For this review, take the finished solid that the model builds, in its own axes (mm). A direction names the side the tool comes from. Round coordinates to 2 decimals unless told otherwise and drop trailing zeros. Loops run counter-clockwise (first coordinate to the right, second up) from the corner with the lowest first, then second, coordinate; pieces in that order, holes last.
```python
from build123d import *

# Parameters (mm, degrees)
EXTRUDE_1_DEPTH      = 38
EXTRUDE_1_DEPTH_BACK = 38
EXTRUDE_2_DEPTH      = 60
SKETCH_4_R           = 1.5
SKETCH_4_W           = 14
SKETCH_4_H           = 18
CUT_EXTRUDE_1_DEPTH  = 6
CUT_EXTRUDE_3_DEPTH  = 14
FILLET_2_R           = 3
CUT_EXTRUDE_6_DEPTH  = 3
SKETCH_13_R          = 1.5
CUT_EXTRUDE_7_DEPTH  = 10
CUT_EXTRUDE_9_DEPTH  = 15
SKETCH_17_W          = 41
SKETCH_17_H          = 26
SKETCH_17_R          = 9.5
SKETCH_17_R_2        = 1.5
EXTRUDE_3_DEPTH      = 3
FILLET_3_R           = 10
SKETCH_18_W          = 17
SKETCH_18_H          = 40
CUT_EXTRUDE_10_DEPTH = 10
FILLET_4_R           = 8
CUT_EXTRUDE_11_DEPTH = 4
FILLET_5_R           = 1
CUT_EXTRUDE_12_DEPTH = 10


with BuildPart() as part:
    # Sketch 2 → Extrude 1 (new, two sides: drawn at the far end of the back side and taken through both)
    with BuildSketch(Plane.XY.offset(-EXTRUDE_1_DEPTH_BACK)):
        Polygon((0, 0), (28.5, 49.363448016), (30.665063509, 48.113448016), (4.618802154, 3), (41, 3), (41, 0), align=None)
    extrude(amount=EXTRUDE_1_DEPTH + EXTRUDE_1_DEPTH_BACK)

    # Sketch 3 → Extrude 2 (add)
    with BuildSketch(Plane.XY.offset(38)):
        Polygon((12.618802154, 16.856406461), (14.118802154, 19.454482672), (23.618802154, 3), (20.618802154, 3), align=None)
    extrude(amount=-EXTRUDE_2_DEPTH)

    # Sketch 4 → Cut-Extrude 1 (cut)
    with BuildSketch(Plane(origin=(0, 0, 0), x_dir=(0, 0, 1), z_dir=(-0.8660254037844365, 0.500000000000004, 0))):
        with Locations(Location((34, 53.25, 0), (0, 0, 270))):
            Circle(SKETCH_4_R)
        with Locations(Location((34, 16.75, 0), (0, 0, 90))):
            Circle(SKETCH_4_R)
        with Locations(Location((-34, 16.75, 0), (0, 0, 270))):
            Circle(SKETCH_4_R)
        with Locations(Location((-34, 53.25, 0), (0, 0, 90))):
            Circle(SKETCH_4_R)
        with Locations((31, 35)):
            Rectangle(SKETCH_4_W, SKETCH_4_H)
        with Locations((-31, 35)):
            Rectangle(SKETCH_4_W, SKETCH_4_H)
    extrude(amount=-CUT_EXTRUDE_1_DEPTH, mode=Mode.SUBTRACT)

    # Sketch 6 → Cut-Extrude 3 (cut)
    with BuildSketch(Plane.XY.offset(38)):
        Polygon((23.618802154, 3), (14.118802154, 19.454482672), (12.618802154, 16.856406461), (20.618802154, 3), align=None)
    extrude(amount=-CUT_EXTRUDE_3_DEPTH, mode=Mode.SUBTRACT)

    # Fillet 2
    fillet_2_edges = [part.edges().sort_by_distance(p)[0] for p in [
        (29.582531755, 48.738448016, 38),
        (29.582531755, 48.738448016, -38),
        (23.082531755, 37.480117767, 38),
        (14.082531755, 21.891660498, 38),
        (14.082531755, 21.891660498, -38),
        (23.082531755, 37.480117767, -38),
    ]]
    fillet(fillet_2_edges, radius=FILLET_2_R)

    # Sketch 11 → Cut-Extrude 6 (cut)
    with BuildSketch(Plane(origin=(19.013139721, 10.977241336, 0), x_dir=(0, 0, -1), z_dir=(0.8660254037844374, 0.5000000000000022, 0))):
        with BuildLine():
            Line((-10, 4), (10, 4))
            ThreePointArc((10, 4), (14, 0), (10, -4))
            Line((10, -4), (-10, -4))
            ThreePointArc((-10, -4), (-14, 0), (-10, 4))
        make_face()
    extrude(amount=-CUT_EXTRUDE_6_DEPTH, mode=Mode.SUBTRACT)

    # Sketch 13 → Cut-Extrude 7 (cut)
    with BuildSketch(Plane(origin=(0, 3, 0), x_dir=(1, 0, 0), z_dir=(0, 1, 0))):
        with Locations(Location((37.5, -27, 0), (0, 0, 270))):
            Circle(SKETCH_13_R)
        with Locations(Location((4, -28, 0), (0, 0, 294.364164798))):
            Circle(SKETCH_13_R)
        with Locations(Location((34, 32, 0), (0, 0, 270))):
            Circle(SKETCH_13_R)
        with Locations(Location((4, 32, 0), (0, 0, 294.364164798))):
            Circle(SKETCH_13_R)
    extrude(amount=-CUT_EXTRUDE_7_DEPTH, mode=Mode.SUBTRACT)

    # Sketch 15 → Cut-Extrude 9 (cut)
    with BuildSketch(Plane.XY.offset(38)):
        Polygon((4.618802154, 3), (1.732050808, 3), (5.196152423, 9), (8.082903769, 9), align=None)
    cut_extrude_9 = extrude(amount=-CUT_EXTRUDE_9_DEPTH, mode=Mode.SUBTRACT)

    # Mirror 1: Cut-Extrude 9 across plane
    add(cut_extrude_9.mirror(Plane.XY), mode=Mode.SUBTRACT)

    # Sketch 17 → Extrude 3 (add)
    # profile 1 of 2: a face of its own
    with BuildSketch(Plane(origin=(0, 3, 0), x_dir=(1, 0, 0), z_dir=(0, 1, 0))):
        with Locations((20.5, 51)):
            Rectangle(SKETCH_17_W, SKETCH_17_H)
        with Locations(Location((17, 50, 0), (0, 0, 270))):
            Circle(SKETCH_17_R, mode=Mode.SUBTRACT)
    # profile 2 of 2: a face of its own
    with BuildSketch(Plane(origin=(0, 3, 0), x_dir=(1, 0, 0), z_dir=(0, 1, 0))):
        with Locations((20.5, -51)):
            Rectangle(SKETCH_17_W, SKETCH_17_H)
        with Locations(Location((5, -45, 0), (0, 0, 270))):
            Circle(SKETCH_17_R_2, mode=Mode.SUBTRACT)
        with Locations(Location((5, -55, 0), (0, 0, 90))):
            Circle(SKETCH_17_R_2, mode=Mode.SUBTRACT)
        with Locations(Location((35, -55, 0), (0, 0, 270))):
            Circle(SKETCH_17_R_2, mode=Mode.SUBTRACT)
        with Locations(Location((35, -45, 0), (0, 0, 90))):
            Circle(SKETCH_17_R_2, mode=Mode.SUBTRACT)
        with Locations(Location((20, -50, 0), (0, 0, 270))):
            Circle(SKETCH_17_R, mode=Mode.SUBTRACT)
    extrude(amount=-EXTRUDE_3_DEPTH)

    # Fillet 3
    fillet_3_edges = [part.edges().sort_by_distance(p)[0] for p in [
        (41, 1.5, -64),
        (0, 1.5, -64),
        (0, 1.5, 64),
        (41, 1.5, 64),
    ]]
    fillet(fillet_3_edges, radius=FILLET_3_R)

    # Sketch 18 → Cut-Extrude 10 (cut)
    with BuildSketch(Plane(origin=(0, 3, 0), x_dir=(1, 0, 0), z_dir=(0, 1, 0))):
        with Locations((32.5, 0)):
            Rectangle(SKETCH_18_W, SKETCH_18_H)
        with BuildLine():
            Line((8, -12.5), (8, 12.5))
            ThreePointArc((8, 12.5), (12, 16.5), (16, 12.5))
            Line((16, 12.5), (16, -12.5))
            ThreePointArc((16, -12.5), (12, -16.5), (8, -12.5))
        make_face()
    extrude(amount=-CUT_EXTRUDE_10_DEPTH, mode=Mode.SUBTRACT)

    # Fillet 4
    fillet_4_edges = [part.edges().sort_by_distance(p)[0] for p in [
        (41, 1.5, -20),
        (41, 1.5, 20),
        (24, 1.5, 20),
        (24, 1.5, -20),
    ]]
    fillet(fillet_4_edges, radius=FILLET_4_R)

    # Sketch 21 → Cut-Extrude 11 (cut)
    with BuildSketch(Plane(origin=(0, 0, 0), x_dir=(0, 0, 1), z_dir=(-0.8660254037844364, 0.5000000000000041, 0))):
        with BuildLine():
            Line((-23.430749028, 57), (23.430749028, 57))
            ThreePointArc((23.430749028, 57), (0, 48), (-23.430749028, 57))
        make_face()
        with BuildLine():
            Line((-8, 19), (8, 19))
            ThreePointArc((8, 19), (12, 15), (8, 11))
            Line((8, 11), (-8, 11))
            ThreePointArc((-8, 11), (-12, 15), (-8, 19))
        make_face()
    extrude(amount=-CUT_EXTRUDE_11_DEPTH, mode=Mode.SUBTRACT)

    # Fillet 5
    fillet_5_edges = [part.edges().sort_by_distance(p)[0] for p in [
        (6.639528096, 9, 23),
        (6.639528096, 9, 38),
        (6.639528096, 9, -38),
        (6.639528096, 9, -23),
        (14.082531755, 21.891660498, 24),
        (23.082531755, 37.480117767, 24),
        (23.082531755, 37.480117767, -24),
        (14.082531755, 21.891660498, -24),
    ]]
    fillet(fillet_5_edges, radius=FILLET_5_R)

    # Sketch 22 → Cut-Extrude 12 (cut)
    with BuildSketch(Plane(origin=(0, 3, 0), x_dir=(1, 0, 0), z_dir=(0, 1, 0))):
        with BuildLine():
            Line((0, -34.931397069), (0, -65.97672588))
            Line((0, -65.97672588), (41, -65.97672588))
            Line((41, -65.97672588), (41, -34.931397069))
            ThreePointArc((41, -34.931397069), (20.5, -40.502499938), (0, -34.931397069))
        make_face()
    extrude(amount=-CUT_EXTRUDE_12_DEPTH, mode=Mode.SUBTRACT)


solid = part.part
```
(1) The part is to be moulded in two halves that separate along Z. For faces 1 (the flat face through (14.07, 21.9, 29.93)), 2 (the cylindrical face through (2.85, 1.48, -60.99)), 3 (the cylindrical face through (9.28, 13.608, 35.464)), 4 (the cylindrical face through (9, 12, 12)), say which applies: pulls with the +Z half, pulls with the -Z half, needs draft (parallel to the pull), parting line crosses it, or undercut.
(2) Insertion check: pin 1 Ø3 at (x, z) = (8, -44) entering from -Y; pin 2 Ø12 at (x, z) = (6, 1.5) entering from +Y; pin 3 Ø0.8 at (x, y) = (32.5, 1.5) entering from -Z; pin 4 Ø3.5 at (y, z) = (1.5, -3.5) entering from +X. Each pin has a flat end and moves straight along its axis. Give the tip position at first contact, or say it passes through.
(3) Add section A-A (z = 2). Give the boundary of the cut face in (x, y).
(4) Add section B-B (z = 18.5). Give the boundary of the cut face in (x, y).
(5) For L1, parallel to X at y = 1, z = 27; L2, parallel to Z at x = 37, y = 2; L3, parallel to X at y = 1, z = -32, list the stretches that pass through material, from the lowest coordinate up.
(6) For faces 5 (the cylindrical face through (4, 1.5, -30.5)), 6 (the cylindrical face through (23.53, 38.21, 37.1)), 7 (the flat face through (19.9, 6.87, -0.14)), list the 3-axis set-ups (+Z, -Z, +X, -X, +Y, -Y) from which the entire face can be reached by the end or side of a thin tool; tool diameter is ignored.
Outcome:
1. face 1: needs draft
1. face 2: pulls with the -Z half
1. face 3: undercut
1. face 4: undercut
2. pin 1: stops at y = 0
2. pin 2: stops at y = 20.78
2. pin 3: stops at z = -63.94
2. pin 4: stops at x = 24
3. outline: (0, 0) - (8, 0) - (8, 3) - (4.62, 3) - (7.67, 8.28) - (5.5, 9.53) - close; (9.5, 16.45) - (11.67, 15.2) - (12.62, 16.86) - (14.76, 13.14) - (17.01, 14.44) - (14.12, 19.45) - (26.19, 40.37) - (24.03, 41.62) - close; (16, 0) - (24, 0) - (24, 3) - (23.62, 3) - (21.01, 7.51) - (18.76, 6.21) - (20.62, 3) - (16, 3) - close
4. outline: (0, 0) - (27.34, 0) - (27.34, 3) - (23.62, 3) - (14.12, 19.45) - (28.81, 44.9) - (26.64, 46.15) - close; hole (4.62, 3) - (20.62, 3) - (12.62, 16.86) - close
5. L1: x = 0.58 to 2.88, 5.12 to 36, 39 to 40.94
5. L2: z = -62 to -21.07, 21.07 to 25.59, 28.41 to 36.99
5. L3: x = 0.58 to 2.5, 5.5 to 32.5, 35.5 to 41
6. face 5: -Y
6. face 6: +Z, -X
6. face 7: none
